Design review of the part built by this model. Coordinates are the model's own, in mm. Round coordinates to 2 decimals unless told otherwise and drop trailing zeros. Loops run counter-clockwise (first coordinate to the right, second up) from the corner with the lowest first, then second, coordinate; pieces in that order, holes last. Notation, with made-up numbers: (9, 74) - (38, 74) arc R35 cw to (38, 107) - close; hole circle Ø1 at (71, -29.5). An arc over 180 degrees is marked (long way). Return JSON: item names as keys, results as strings. Group by question number.
(1) We need section C-C, the plane x = 56. Write out the cut boundary in (y, z).
(2) Clearance check with flat-ended pins moving along their axes: pin 1 (1.6 mm diameter, centred on x = 18.5, z = 5, fed in from +Y); pin 2 (15 mm diameter, centred on x = 26, y = -26, fed in from +Z); pin 3 (10 mm diameter, centred on y = 10.5, z = 10.5, fed in from -X); pin 4 (3 mm diameter, centred on x = 26, y = -23, fed in from +Z). State where each tip first meets the part, or that it passes through.
(3) We need section A-A, the plane z = 24.5. Write out the cut boundary in (x, y), and give its area (3 significant figures).
(4) Wall thickness on L1, parallel to Z at x = 49, y = 12: over which ranges is the line inside the solid? List them lowest first. Write a range as [from, to].
(5) We need section B-B, the plane y = 6. Write out the cut boundary in (x, z), and give its area (3 significant figures).
Autodesk Fusion 360 part; units mm, degrees
sketch "Sketch1" plane through (0, 0, 0) normal (0, 0, 1) x (1, 0, 0)
  line L0 (-44.8667, 47.2814) -> (95.1333, 47.2814)
  line L1 (95.1333, 47.2814) -> (95.1333, -92.7186)
  line L2 (95.1333, -92.7186) -> (-44.8667, -92.7186)
  line L3 (-44.8667, -92.7186) -> (-44.8667, 47.2814)
  dimension "d1" = 140
  dimension "d2" = 140
extrude "Extrude1" add sketch "Sketch1" along normal blind 3
sketch "Sketch2" plane through (0, 0, 3) normal (0, 0, 1) x (-1, 0, 0)
  line L0 (44.8667, 92.7186) -> (-95.1333, 92.7186)
  line L1 (-95.1333, 92.7186) -> (-95.1333, -47.2814)
  line L2 (-95.1333, -47.2814) -> (44.8667, -47.2814)
  line L3 (44.8667, -47.2814) -> (44.8667, 92.7186)
  line L4 (44.8667, -47.2814) -> (39.8667, -47.2814)
  line L5 (39.8667, -47.2814) -> (39.8667, -42.2814)
  line L6 (39.8667, -42.2814) -> (44.8667, -42.2814)
  line L7 (44.8667, -42.2814) -> (44.8667, -47.2814)
  line L8 (44.8667, 92.7186) -> (39.8667, 92.7186)
  line L9 (39.8667, 92.7186) -> (39.8667, 87.7186)
  line L10 (39.8667, 87.7186) -> (44.8667, 87.7186)
  line L11 (44.8667, 87.7186) -> (44.8667, 92.7186)
  line L12 (-95.1333, 92.7186) -> (-90.1333, 92.7186)
  line L13 (-90.1333, 92.7186) -> (-90.1333, 87.7186)
  line L14 (-90.1333, 87.7186) -> (-95.1333, 87.7186)
  line L15 (-95.1333, 87.7186) -> (-95.1333, 92.7186)
  line L16 (-95.1333, -47.2814) -> (-90.1333, -47.2814)
  line L17 (-90.1333, -47.2814) -> (-90.1333, -42.2814)
  line L18 (-90.1333, -42.2814) -> (-95.1333, -42.2814)
  line L19 (-95.1333, -42.2814) -> (-95.1333, -47.2814)
  dimension "d5" = 5
  dimension "d6" = 5
  dimension "d7" = 5
  dimension "d8" = 5
  dimension "d9" = 5
  dimension "d10" = 5
  dimension "d11" = 5
  dimension "d12" = 5
extrude "Extrude2" add sketch "Sketch2" along normal blind 48 contours L0 L3 L8 L9 L10 L11 | L0 L1 L12 L13 L14 L15 | L2 L3 L4 L5 L6 L7 | L1 L2 L16 L17 L18 L19
sketch "Sketch3" plane through (0, 0, 3) normal (0, 0, 1) x (-1, 0, 0)
  line L0 (-90.1333, 92.7186) -> (-90.1333, 87.7186)
  line L1 (-90.1333, 87.7186) -> (-95.1333, 87.7186)
  line L2 (-95.1333, 87.7186) -> (-95.1333, -42.2814)
  line L3 (-95.1333, -42.2814) -> (-90.1333, -42.2814)
  line L4 (-90.1333, -42.2814) -> (-90.1333, -47.2814)
  line L5 (-90.1333, -47.2814) -> (39.8667, -47.2814)
  line L6 (39.8667, -47.2814) -> (39.8667, -42.2814)
  line L7 (39.8667, -42.2814) -> (44.8667, -42.2814)
  line L8 (44.8667, -42.2814) -> (44.8667, 87.7186)
  line L9 (44.8667, 87.7186) -> (39.8667, 87.7186)
  line L10 (39.8667, 87.7186) -> (39.8667, 92.7186)
  line L11 (39.8667, 92.7186) -> (-90.1333, 92.7186)
  circle A0 centre (-25.1333, 22.7186) radius 2
  line L12 (-27.1333, 31.4686) -> (-23.1333, 31.4686)
  line L13 (-23.1333, 31.4686) -> (-23.1333, 13.9686)
  line L14 (-23.1333, 13.9686) -> (-27.1333, 13.9686)
  line L15 (-27.1333, 13.9686) -> (-27.1333, 31.4686)
  line L16 (-33.8833, 24.7186) -> (-16.3833, 24.7186)
  line L17 (-16.3833, 24.7186) -> (-16.3833, 20.7186)
  line L18 (-16.3833, 20.7186) -> (-33.8833, 20.7186)
  line L19 (-33.8833, 20.7186) -> (-33.8833, 24.7186)
  dimension "d15" = 4
  dimension "d16" = 70
  dimension "d17" = 70
  dimension "d18" = 4
  dimension "d19" = 17.5
  dimension "d20" = 8.75
  dimension "d21" = 2
  dimension "d22" = 17.5
  dimension "d23" = 4
  dimension "d24" = 2
  dimension "d25" = 8.75
extrude "Extrude3" add sketch "Sketch3" along normal blind 3.3 contours A0 L13 L18 | A0 L13 L16 | L13 L16 L17 L18 | A0 L15 L16 | L12 L13 L15 L16 | A0 L15 L18 | L13 L14 L15 L18 | L15 L16 L18 L19
sketch "Sketch4" plane through (0, 0, 6.3) normal (0, 0, 1) x (-1, 0, 0)
  circle A0 centre (-25.1333, 22.7186) radius 2
  line L0 (-33.8833, 20.7186) -> (-27.1333, 20.7186)
  line L1 (-27.1333, 20.7186) -> (-27.1333, 13.9686)
  line L2 (-27.1333, 13.9686) -> (-23.1333, 13.9686)
  line L3 (-23.1333, 13.9686) -> (-23.1333, 20.7186)
  line L4 (-23.1333, 20.7186) -> (-16.3833, 20.7186)
  line L5 (-16.3833, 20.7186) -> (-16.3833, 24.7186)
  line L6 (-16.3833, 24.7186) -> (-23.1333, 24.7186)
  line L7 (-23.1333, 24.7186) -> (-23.1333, 31.4686)
  line L8 (-23.1333, 31.4686) -> (-27.1333, 31.4686)
  line L9 (-27.1333, 31.4686) -> (-27.1333, 24.7186)
  line L10 (-27.1333, 24.7186) -> (-33.8833, 24.7186)
  line L11 (-33.8833, 24.7186) -> (-33.8833, 20.7186)
  line L12 (-27.1333, 31.4686) -> (-23.1333, 31.4686)
  line L13 (-23.1333, 31.4686) -> (-23.1333, 29.4686)
  line L14 (-23.1333, 29.4686) -> (-27.1333, 29.4686)
  line L15 (-27.1333, 29.4686) -> (-27.1333, 31.4686)
  line L16 (-16.3833, 24.7186) -> (-18.3833, 24.7186)
  line L17 (-18.3833, 24.7186) -> (-18.3833, 20.7186)
  line L18 (-18.3833, 20.7186) -> (-16.3833, 20.7186)
  line L19 (-16.3833, 20.7186) -> (-16.3833, 24.7186)
  line L20 (-23.1333, 13.9686) -> (-27.1333, 13.9686)
  line L21 (-27.1333, 13.9686) -> (-27.1333, 15.9686)
  line L22 (-27.1333, 15.9686) -> (-23.1333, 15.9686)
  line L23 (-23.1333, 15.9686) -> (-23.1333, 13.9686)
  line L24 (-33.8833, 24.7186) -> (-31.8833, 24.7186)
  line L25 (-31.8833, 24.7186) -> (-31.8833, 20.7186)
  line L26 (-31.8833, 20.7186) -> (-33.8833, 20.7186)
  line L27 (-33.8833, 20.7186) -> (-33.8833, 24.7186)
  dimension "d28" = 2
  dimension "d29" = 2
  dimension "d30" = 4
  dimension "d31" = 4
  dimension "d32" = 2
  dimension "d33" = 2
  dimension "d34" = 4
  dimension "d40" = 4
extrude "Extrude4" add sketch "Sketch4" along normal blind 2 contours L0 L10 L11 L24 L25 L26 L27 | L1 L2 L3 L20 L21 L22 L23 | L7 L8 L9 L12 L13 L14 L15 | L4 L5 L6 L16 L17 L18 L19
sketch "Sketch5" plane through (0, 0, 6.3) normal (0, 0, 1) x (-1, 0, 0)
  line L0 (-18.3833, 20.7186) -> (-18.3833, 24.7186)
  line L1 (-18.3833, 24.7186) -> (-23.1333, 24.7186)
  line L2 (-23.1333, 24.7186) -> (-23.1333, 29.4686)
  line L3 (-27.1333, 29.4686) -> (-27.1333, 24.7186)
  line L4 (-27.1333, 24.7186) -> (-31.8833, 24.7186)
  line L5 (-31.8833, 24.7186) -> (-31.8833, 20.7186)
  line L6 (-31.8833, 20.7186) -> (-27.1333, 20.7186)
  line L7 (-27.1333, 20.7186) -> (-27.1333, 15.9686)
  line L8 (-27.1333, 15.9686) -> (-23.1333, 15.9686)
  line L9 (-23.1333, 15.9686) -> (-23.1333, 20.7186)
  line L10 (-23.1333, 20.7186) -> (-18.3833, 20.7186)
  circle A0 centre (-25.1333, 22.7186) radius 2
  circle A1 centre (-25.1333, 22.7186) radius 16
  line L11 (-23.1333, 29.4686) -> (-27.1333, 29.4686)
  dimension "d37" = 32
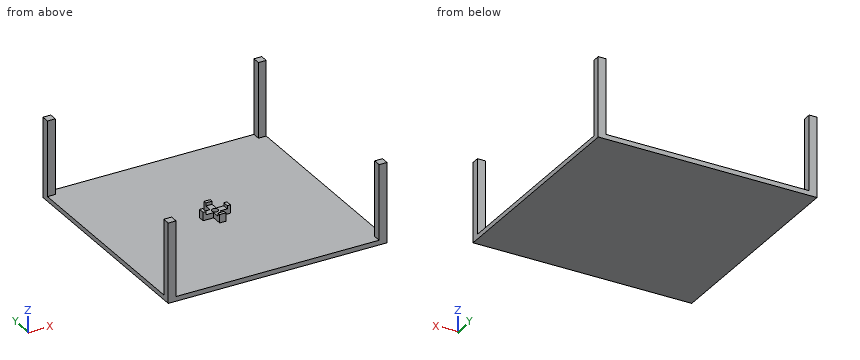
Solutions:
{
 "1": {"outline": "(-92.72, 0) - (47.28, 0) - (47.28, 3) - (-92.72, 3) - close"},
 "2": {"pin 1": "y = -20.72", "pin 2": "z = 8.3", "pin 3": "through", "pin 4": "z = 6.3"},
 "3": {"outline": "(-44.87, -92.72) - (-39.87, -92.72) - (-39.87, -87.72) - (-44.87, -87.72) - close; (-44.87, 42.28) - (-39.87, 42.28) - (-39.87, 47.28) - (-44.87, 47.28) - close; (90.13, -92.72) - (95.13, -92.72) - (95.13, -87.72) - (90.13, -87.72) - close; (90.13, 42.28) - (95.13, 42.28) - (95.13, 47.28) - (90.13, 47.28) - close", "area": "100 mm^2"},
 "4": {"L1": "[0, 3]"},
 "5": {"outline": "(-44.87, 0) - (95.13, 0) - (95.13, 3) - (-44.87, 3) - close", "area": "420 mm^2"}
}
